Autodesk Inventor part; units mm, degrees
ref_plane "YZ Plane" through (0, 0, 0) normal (1, 0, 0) x (0, 1, 0)
ref_plane "XZ Plane" through (0, 0, 0) normal (0, 1, 0) x (-1, 0, 0)
ref_plane "XY Plane" through (0, 0, 0) normal (0, 0, 1) x (1, 0, 0)
sketch "Sketch1" plane through (0, 0, 0) normal (0, 0, 1) x (1, 0, 0)
  line L0 (0, 0) -> (72.4, 0)
  line L1 (72.4, 0) -> (72.4, 71)
  line L2 (72.4, 71) -> (0, 71)
  line L3 (0, 71) -> (0, 0)
  dimension "d0" = 72.4
  dimension "d1" = 71
extrude "Extrusion1" add sketch "Sketch1" along normal blind 10
sketch "Sketch2" plane through (0, 0, 10) normal (0, 0, 1) x (1, 0, 0)
  line L0 (72.4, 0) -> (72.4, 71)
  line L1 (72.4, 15.5) -> (82.4, 15.5)
  line L2 (82.4, 15.5) -> (82.4, 55.5)
  line L3 (82.4, 55.5) -> (72.4, 55.5)
  line L4 (72.4, 55.5) -> (72.4, 15.5)
  line L5 (72.4, 71) -> (0, 71)
  circle A0 centre (77.4, 35.5) radius 2.5
  line L6 (0, 0) -> (72.4, 0)
  point P0 (82.4, 35.5)
  point P1 (77.4, 55.5)
  dimension "d4" = 10
  dimension "d5" = 40
  dimension "d7" = 5
  dimension "d31" = 15.5
extrude "Extrusion2" add sketch "Sketch2" against normal blind 10
sketch "Sketch3" plane through (0, 0, 10) normal (0, 0, 1) x (1, 0, 0)
  line L0 (72.4, 55.5) -> (82.4, 55.5)
  line L1 (72.4, 15.5) -> (82.4, 15.5)
  line L2 (82.4, 55.5) -> (72.4, 55.5)
  line L3 (72.4, 55.5) -> (72.4, 15.5)
  line L4 (72.4, 15.5) -> (82.4, 15.5)
  line L5 (82.4, 15.5) -> (82.4, 55.5)
  point P0 (0, 0)
extrude "Extrusion3" cut sketch "Sketch3" against normal blind 5
sketch "Sketch4" plane through (0, 0, 0) normal (0, 0, -1) x (-1, 0, 0)
  line L0 (0, 71) -> (0, 0)
  line L1 (0, 55.5) -> (-10, 55.5)
  line L2 (-10, 55.5) -> (-10, 15.5)
  line L3 (-10, 15.5) -> (0, 15.5)
  line L4 (0, 15.5) -> (0, 55.5)
  point P0 (-72.4, 55.5)
  dimension "d15" = 10
  dimension "d16" = 40
extrude "Extrusion4" cut sketch "Sketch4" against normal blind 5
sketch "Sketch5" plane through (0, 0, 5) normal (0, 0, -1) x (-1, 0, 0)
  circle A0 centre (-5, 35.5) radius 2.5
  line L0 (0, 55.5) -> (0, 15.5)
  line L1 (-10, 55.5) -> (0, 55.5)
  point P0 (0, 0)
  point P1 (0, 35.5)
  point P2 (-5, 55.5)
  dimension "d19" = 5
extrude "Extrusion5" cut sketch "Sketch5" against normal through all
sketch "Sketch8" plane through (0, 0, 0) normal (0, 0, -1) x (-1, 0, 0)
  line L0 (-12.4, 10) -> (-52.4, 10)
  line L1 (-52.4, 10) -> (-52.4, 0)
  line L2 (-52.4, 0) -> (-12.4, 0)
  line L3 (-12.4, 0) -> (-12.4, 10)
  line L4 (0, 0) -> (-72.4, 0)
  line L5 (-72.4, 0) -> (-72.4, 15.5)
  point P0 (-36.2, 0)
  dimension "d32" = 40
  dimension "d33" = 10
  dimension "d34" = 20
extrude "Extrusion8" cut sketch "Sketch8" against normal blind 5
sketch "Sketch9" plane through (0, 0, 5) normal (0, 0, -1) x (-1, 0, 0)
  line L0 (-52.4, 10) -> (-12.4, 10) construction
  line L1 (-52.4, 0) -> (-52.4, 10) construction
  line L2 (-12.4, 0) -> (-52.4, 0) construction
  line L3 (-12.4, 10) -> (-12.4, 0) construction
  circle A0 centre (-32.4, 5) radius 2.5
  point P0 (0, 0)
  point P1 (-32.4, 0)
  point P2 (-12.4, 5)
  dimension "d37" = 5
extrude "Extrusion9" cut sketch "Sketch9" against normal through all
properties part number "SP002" material "ABS Plastic"
Build history of the part. All positions in model axes, mm. A direction names the side the tool comes from. Coordinates: 2 decimals unless noted, no trailing zeros. Write each loop counter-clockwise with the first axis right and the second up, starting at its lowest first coordinate (ties: lowest second). Pieces come first, ordered by that corner, then holes.
(1) 3-axis set-ups, long thin cutter, end or side, ignore diameter. For faces 1 (the flat face through (12.4, 5, 2)), 2 (the flat face through (5, 55.5, 2)), 3 (the flat face through (74, 36, 5)): which of +Z, -Z, +X, -X, +Y, -Y reach the whole face in a straight line?
(2) Mould opens along X. For faces 4 (the flat face through (0, 36, 6)), 5 (the cylindrical face through (74.9, 35.6, 2.5)), 6 (the flat face through (41, 36, 0)) say: pulls with the +X half, pulls with the -X half, needs draft (parallel to the pull), parting line crosses it, or undercut.
(3) Pin check, flat tips, straight feed: pin 1 Ø2.5 at (x, z) = (7, 1.5) entering from -Y; pin 2 Ø4 at (x, y) = (77.4, 35.5) entering from +Z; pin 3 Ø1.5 at (x, z) = (79, 3) entering from -Y; pin 4 Ø1.5 at (y, z) = (5.5, 3) entering from +X. Stop position of each tip, or through.
(4) Drill centre lines: line 1 (Y direction, x = 4.5, z = 1.5); line 2 (Y direction, x = 5, z = 7.95); line 3 (X direction, y = 28, z = 4.5). Where is each one in solid material? Low to high.
(5) Cut at D-D on z = 1.25. List the corners of the cut face in (x, y), and give its area (3 significant figures).
(6) Cut at B-B on x = 32.4. List the corners of the cut face in (y, z), and give its area (3 significant figures).
(7) Cut at A-A on y = 35.5. List the corners of the cut face in (x, z).
(8) Cut at C-C on z = 7.25. List the corners of the cut face in (x, y), and give its area (3 significant figures).
Working result:
1. face 1: -Z, -Y
1. face 2: -Z, -X
1. face 3: +Z, +X, +Y, -Y
2. face 4: pulls with the -X half
2. face 5: undercut
2. face 6: needs draft
3. pin 1: stops at y = 0
3. pin 2: passes through
3. pin 3: stops at y = 15.5
3. pin 4: stops at x = 72.4
4. line 1: y = 0 to 15.5, 55.5 to 71
4. line 2: y = 0 to 33, 38 to 71
4. line 3: x = 10 to 82.4
5. outline: (0, 0) - (12.4, 0) - (12.4, 10) - (52.4, 10) - (52.4, 0) - (72.4, 0) - (72.4, 15.5) - (82.4, 15.5) - (82.4, 55.5) - (72.4, 55.5) - (72.4, 71) - (0, 71) - (0, 55.5) - (10, 55.5) - (10, 15.5) - (0, 15.5) - close; hole circle Ø5 at (77.4, 35.5)
5. area: 4,720 mm2
6. outline: (0, 5) - (2.5, 5) - (2.5, 10) - (0, 10) - close; (7.5, 5) - (10, 5) - (10, 0) - (71, 0) - (71, 10) - (7.5, 10) - close
6. area: 635 mm2
7. outline: (0, 5) - (2.5, 5) - (2.5, 10) - (0, 10) - close; (7.5, 5) - (10, 5) - (10, 0) - (74.9, 0) - (74.9, 5) - (72.4, 5) - (72.4, 10) - (7.5, 10) - close; (79.9, 0) - (82.4, 0) - (82.4, 5) - (79.9, 5) - close
8. outline: (0, 0) - (72.4, 0) - (72.4, 71) - (0, 71) - close; hole circle Ø5 at (5, 35.5); hole circle Ø5 at (32.4, 5)
8. area: 5,100 mm2
